from build123d import *

# Parameters (mm, degrees)
EXTRUDE_1_DEPTH     = 8
SKETCH_3_W          = 20
SKETCH_3_H          = 4
EXTRUDE_2_DEPTH     = 1
SKETCH_4_R          = 2.25
CUT_EXTRUDE_3_DEPTH = 10
CHAMFER_2_SIZE      = 1
CHAMFER_3_SIZE      = 2
CHAMFER_4_SIZE      = 2
SKETCH_6_W          = 20
SKETCH_6_H          = 8
EXTRUDE_3_DEPTH     = 8
SKETCH_7_W          = 10
SKETCH_7_H          = 21
CUT_EXTRUDE_4_DEPTH = 54.833075335
FILLET_1_R          = 2
SKETCH_8_R          = 2.4
CUT_EXTRUDE_5_DEPTH = 6
SKETCH_9_W          = 5
SKETCH_9_H          = 8
EXTRUDE_4_DEPTH     = 16
CHAMFER_5_SIZE      = 2
CHAMFER_6_SIZE      = 2


# Some blends are built 0.0001 mm under size
with BuildPart() as part:
    # ｽｹｯﾁ1 → ﾎﾞｽ - 押し出し1 (new body)
    with BuildSketch(Plane.XY):
        Polygon((-10, 0), (0, 0), (10, 0), (10, 5), (0, 5), (-10, 5), align=None)
        Polygon((0, 5), (10, 5), (10, 39), (-10, 39), (-10, 5), align=None)
        Polygon((-10, 39), (10, 39), (25, 39), (25, 47), (-25, 47), (-25, 39), align=None)
    extrude(amount=-EXTRUDE_1_DEPTH)

    # ｽｹｯﾁ3 → ﾎﾞｽ - 押し出し2 (add)
    with BuildSketch(Plane.XY):
        with Locations((0, 37)):
            Rectangle(SKETCH_3_W, SKETCH_3_H)
    extrude(amount=EXTRUDE_2_DEPTH)

    # ｽｹｯﾁ4 → ｶｯﾄ - 押し出し3 (cut)
    with BuildSketch(Plane(origin=(0, 47, 0), x_dir=(1, 0, 0), z_dir=(0, 1, 0))):
        with Locations(Location((19, 3.847406514, 0), (0, 0, 180))):
            Circle(SKETCH_4_R)
        with Locations(Location((-19, 3.847406514, 0), (0, 0, 180))):
            Circle(SKETCH_4_R)
    extrude(amount=-CUT_EXTRUDE_3_DEPTH, mode=Mode.SUBTRACT)

    # 面取り2
    chamfer_2_edges = [part.edges().sort_by_distance(p)[0] for p in [
        (0, 47, 0),
    ]]
    chamfer(chamfer_2_edges, length=CHAMFER_2_SIZE)

    # 面取り3
    chamfer_3_edges = [part.edges().sort_by_distance(p)[0] for p in [
        (-10, 39, -4),
        (10, 39, -4),
    ]]
    chamfer(chamfer_3_edges, length=CHAMFER_3_SIZE)

    # 面取り4
    # the kernel refuses this chamfer: 2 mm, written as the material it adds along each edge
    with BuildSketch(Plane(origin=(10, 35, 0), x_dir=(0, -0.9996219169112968, -0.02749587661058639), z_dir=(-1, 0, 0))) as chamfer_4_piece_1_section:
        Polygon((CHAMFER_4_SIZE * 0.999621916911, CHAMFER_4_SIZE * 0.0274958766106), (-CHAMFER_4_SIZE * 0.0274958766106, CHAMFER_4_SIZE * 0.999621916911), (0, 0), align=None)
    chamfer_4_piece_1 = extrude(amount=20, mode=Mode.PRIVATE)
    chamfer_4_piece_1 = split(chamfer_4_piece_1, bisect_by=Plane(origin=(0, 34.213197832, 1), z_dir=(0, 0, -1)), keep=Keep.TOP, mode=Mode.PRIVATE)
    add(chamfer_4_piece_1)

    # ｽｹｯﾁ6 → ﾎﾞｽ - 押し出し3 (add)
    with BuildSketch(Plane.XY):
        with Locations((0, 4)):
            Rectangle(SKETCH_6_W, SKETCH_6_H)
    extrude(amount=EXTRUDE_3_DEPTH)

    # ｽｹｯﾁ7 → ｶｯﾄ - 押し出し4 (cut, through all)
    with BuildSketch(Plane.XY):
        with Locations((0, 20.5)):
            Rectangle(SKETCH_7_W, SKETCH_7_H)
    extrude(amount=-CUT_EXTRUDE_4_DEPTH, mode=Mode.SUBTRACT)

    # ﾌｨﾚｯﾄ1
    fillet_1_edges = [part.edges().sort_by_distance(p)[0] for p in [
        (5, 31, -4),
        (5, 10, -4),
        (-5, 10, -4),
        (-5, 31, -4),
    ]]
    fillet(fillet_1_edges, radius=FILLET_1_R)

    # ｽｹｯﾁ8 → ｶｯﾄ - 押し出し5 (cut)
    with BuildSketch(Plane.XZ):
        with Locations(Location((-6, 0, 0), (0, 0, 270))):
            Circle(SKETCH_8_R)
        with Locations(Location((6, 0, 0), (0, 0, 270))):
            Circle(SKETCH_8_R)
    extrude(amount=-CUT_EXTRUDE_5_DEPTH, mode=Mode.SUBTRACT)

    # ｽｹｯﾁ9 → ﾎﾞｽ - 押し出し4 (add)
    with BuildSketch(Plane.XY.offset(8)):
        with Locations((12.5, 4)):
            Rectangle(SKETCH_9_W, SKETCH_9_H)
        with Locations((-12.5, 4)):
            Rectangle(SKETCH_9_W, SKETCH_9_H)
    extrude(amount=-EXTRUDE_4_DEPTH)

    # 面取り5
    chamfer_5_edges = [part.edges().sort_by_distance(p)[0] for p in [
        (0, 8, 8),
    ]]
    chamfer(chamfer_5_edges, length=CHAMFER_5_SIZE)

    # 面取り6
    chamfer_6_edges = [part.edges().sort_by_distance(p)[0] for p in [
        (0, 8, 0),
        (10, 8, -4),
        (-10, 8, -4),
    ]]
    chamfer(chamfer_6_edges, length=CHAMFER_6_SIZE - 0.0001)  # a hair under: the kernel refuses the full size


solid = part.part
Here's how the part is built. I have some questions about the finished solid (model axes, mm). A direction names the side the tool comes from. Give positions to 0.01 mm unless a question says otherwise; leave off trailing zeros. Order: outer loops, then holes, each group sorted by start corner. A loop starts at its lowest first (then second) coordinate and runs counter-clockwise, first axis right, second up. Notation, with made-up numbers: M 89,4.5 L 125,4.5 A18 cw 125,12.5 Z; hole C 68.5,75 d9. An arc over 180 degrees is marked long. Answer as a JSON object with one key per item and string values. Group by question number.
1) Suppose I cut it at A-A, the plane x = -19. Write out the boundary of the cut face in (y, z), plus the area to 3 significant figures.
2) On a 3-axis mill with a long thin cutter (end or side, diameter ignored), from which of +Z, -Z, +X, -X, +Y, -Y can I reach the whole of each face in a straight line? I mean faces 1 (the flat face through (-15, 4, 0)), 2 (the flat face through (-17, 39, -6)), 3 (the cylindrical face through (-3.62, 2.96, 0.31)), 4 (the flat face through (5, 20, -4)). Say none if no direction works.
3) I'm going to push flat-ended pins straight in: pin 1 Ø7 at (x, z) = (19, -3.85) entering from +Y; pin 2 Ø1.4 at (x, z) = (-6, 0) entering from -Y; pin 3 Ø1.1 at (x, z) = (5, 0.5) entering from +Y; pin 4 Ø7 at (x, y) = (1.5, 41) entering from +Z. Where does each tip first touch, or does it pass through?
4) We'd pull the mould along Y, two halves only. Please class faces 5 (the flat face through (10, 24, -4)), 6 (the flat face through (0, 7, 7)), 7 (the cylindrical face through (-21.146, 43.056, -3.172)), 8 (the flat face through (-6, 6, 0)): pulls with the +Y half, pulls with the -Y half, needs draft (parallel to the pull), parting line crosses it, or undercut.
5) Please list where these lines run through material, in increasing order: L1, parallel to X at y = 4.7, z = 0; L2, parallel to X at y = 19.5, z = -5; L3, parallel to Z at x = 19, y = 43.25. Write a range as [from, to].
6) Suppose I cut it at B-B, the plane y = 22.5. Write out the boundary of the cut face in (x, z).
7) Suppose I cut it at D-D, the plane x = -6. Write out the boundary of the cut face in (y, z).
Results found:
{
 "1": {"outline": "M 39,-8 L 47,-8 L 47,-6.1 L 39,-6.1 Z; M 39,-1.6 L 47,-1.6 L 47,-1 L 46,0 L 39,0 Z", "area": "27.5 mm²"},
 "2": {"face 1": "+Z, -Z, -X, -Y", "face 2": "+Z, -Z, -X", "face 3": "-Y", "face 4": "+Z, -Z"},
 "3": {"pin 1": "y = 47", "pin 2": "y = 6", "pin 3": "y = 46.05", "pin 4": "z = 1"},
 "4": {"face 5": "undercut", "face 6": "pulls with the +Y half", "face 7": "needs draft", "face 8": "pulls with the -Y half"},
 "5": {"L1": "[-15, -8.4], [-3.6, 3.6], [8.4, 15]", "L2": "[-10, -5], [5, 10]", "L3": "[-8, -6.1], [-1.6, 0]"},
 "6": {"outline": "M -10,-8 L -5,-8 L -5,0 L -10,0 Z; M 5,-8 L 10,-8 L 10,0 L 5,0 Z"},
 "7": {"outline": "M 0,-8 L 47,-8 L 47,-1 L 46,0 L 39,0 L 39,1 L 34,1 L 33,0 L 10,0 L 8,2 L 8,6 L 6,8 L 0,8 L 0,2.4 L 6,2.4 L 6,-2.4 L 0,-2.4 Z"}
}
